Autodesk Inventor part; units mm, degrees
ref_plane "YZ Plane" through (0, 0, 0) normal (1, 0, 0) x (0, 1, 0)
ref_plane "XZ Plane" through (0, 0, 0) normal (0, 1, 0) x (-1, 0, 0)
ref_plane "XY Plane" through (0, 0, 0) normal (0, 0, 1) x (1, 0, 0)
sketch "Sketch1" plane through (0, 0, 0) normal (0, 0, 1) x (1, 0, 0)
  line L0 (32.5, 60) -> (-32.5, 60)
  line L1 (-32.5, 60) -> (-32.5, -60)
  line L2 (-32.5, -60) -> (32.5, -60)
  line L3 (32.5, -60) -> (32.5, 60)
  line L4 (32.5, 60) -> (-32.5, -60) construction
  line L5 (-32.5, 60) -> (32.5, -60) construction
  line L6 (-27, 57) -> (27, 57) construction
  line L7 (27, 57) -> (27, -57) construction
  line L8 (27, -57) -> (-27, -57) construction
  line L9 (-27, -57) -> (-27, 57) construction
  line L10 (-27, 57) -> (27, -57) construction
  line L11 (27, 57) -> (-27, -57) construction
  arc A0 (22.4174, 59) -> (31.5, 54.8206) centre (27, 57) ccw
  line L12 (31.5, 54.8206) -> (31.5, -54.8206)
  line L13 (22.4174, 59) -> (-22.4174, 59)
  line L14 (32.5, 0) -> (-32.5, 0) construction
  line L15 (0, 60) -> (0, -60) construction
  arc A1 (31.5, -54.8206) -> (22.4174, -59) centre (27, -57) ccw
  line L16 (22.4174, -59) -> (-22.4174, -59)
  arc A2 (-31.5, 54.8206) -> (-22.4174, 59) centre (-27, 57) ccw
  line L17 (-31.5, 54.8206) -> (-31.5, -54.8206)
  arc A3 (-22.4174, -59) -> (-31.5, -54.8206) centre (-27, -57) ccw
  point P0 (0, 0)
  dimension "d0" = 65
  dimension "d1" = 120
  dimension "d2" = 5.5
  dimension "d3" = 3
  dimension "d4" = 1
  dimension "d5" = 1
  dimension "d6" = 5
extrude "Extrusion1" add sketch "Sketch1" along normal blind 1.6 contours L3 L2 L1 L0 | A0 L12 A1 L16 A3 L17 A2 L13
extrude "Extrusion2" add sketch "Sketch1" along normal blind 14.1 contours A0 L12 A1 L16 A3 L17 A2 L13
hole "Hole1" at (27, 57, 0) at (-27, 57, 0) at (-27, -57, 0) at (27, -57, 0) direction (0, 0, 1) diameter 3.5 end through all
fillet "Fillet1" radius 2 8 edges at (-22.4174, 59, 7.85) (-31.5, 54.8206, 7.85) (22.4174, 59, 7.85) (31.5, 54.8206, 7.85) (31.5, -54.8206, 7.85) (22.4174, -59, 7.85) (-22.4174, -59, 7.85) (-31.5, -54.8206, 7.85)
equation "\"d5\" = d4"
properties part number "SUSTAINA-CORE-BOARD" material "Acetal Resin, Black"
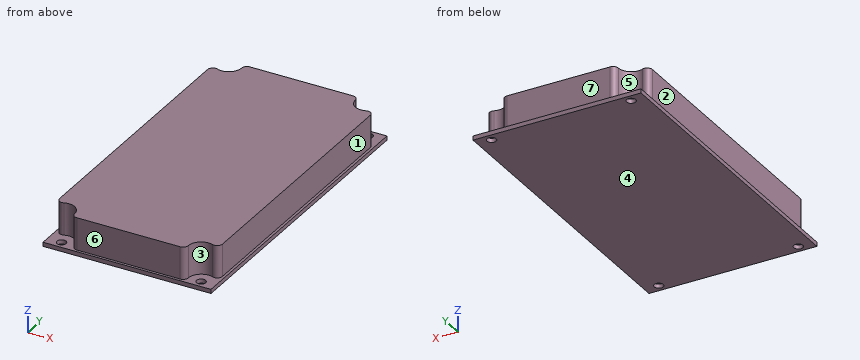
Verification items for the finished model (mm, model axes). Face numbers are marked on the shaded views. A direction names the side the tool comes from. Give positions to 0.01 mm unless a question says otherwise; leave off trailing zeros. Write each loop counter-clockwise with the first axis right and the second up, starting at its lowest first coordinate (ties: lowest second). Pieces come first, ordered by that corner, then holes. Notation, with made-up numbers: M 25.25,26.25 L 77.25,26.25 A10 cw 77.25,33.25 Z; hole C 55,9.25 d8. An arc over 180 degrees is marked long. Use CSV: the item, a comma, the result in double quotes.
1) Release check for a two-part mould opening along X. For the marked faces 1, 2 and 3 record: released by +X, released by -X, zero draft, split by the parting line, or undercut.
Final values:
face 1,"released by +X"
face 2,"released by -X"
face 3,"undercut"
2) Cross-section at A-A (x = -27). Enter the section's corners in (y, z).
Final values:
outline,"M -60,0 L -58.75,0 L -58.75,1.6 L -60,1.6 Z; M -55.25,0 L 55.25,0 L 55.25,1.6 L 52,1.6 L 52,14.1 L -52,14.1 L -52,1.6 L -55.25,1.6 Z; M 58.75,0 L 60,0 L 60,1.6 L 58.75,1.6 Z"
3) Cross-section at B-B (y = 35). Enter the section's corners in (x, z), plus the area to 4 significant figures.
Final values:
outline,"M -32.5,0 L 32.5,0 L 32.5,1.6 L 31.5,1.6 L 31.5,14.1 L -31.5,14.1 L -31.5,1.6 L -32.5,1.6 Z"
area,"891.5 mm²"
4) Go/stop test with flat-tipped pins: pin 1 Ø6 at (y, z) = (45.5, 11) entering from +X; pin 2 Ø5.5 at (x, y) = (-27, -57) entering from +Z; pin 3 Ø1.5 at (x, z) = (9, 11) entering from -Y. Record where each tip stops, or that it passes through.
Final values:
pin 1,"x = 31.5"
pin 2,"z = 1.6"
pin 3,"y = -59"
5) Cross-section at C-C (z = 12.25). Enter the section's corners in (x, y), plus the area to 3 significant figures.
Final values:
outline,"M -31.5,-50.46 A2 ccw -28.79,-52.33 A5 cw -22,-57 A2 ccw -20,-59 L 20,-59 A2 ccw 22,-57 A5 cw 28.79,-52.33 A2 ccw 31.5,-50.46 L 31.5,50.46 A2 ccw 28.79,52.33 A5 cw 22,57 A2 ccw 20,59 L -20,59 A2 ccw -22,57 A5 cw -28.79,52.33 A2 ccw -31.5,50.46 Z"
area,"7,190 mm²"
6) Access from +Z, -Z, +X, -X, +Y, -Y to the whole of each face (thin tool, end or side, straight path). Record for the marked faces 4, 5, 6 and 7.
Final values:
face 4,"-Z, +X, -X, +Y, -Y"
face 5,"+Z, +Y"
face 6,"+Z, +X, -X, -Y"
face 7,"+Z, +X, -X, +Y"
7) Material ranges on line 1 along Y through (x, z) = (-27, 0.8); line 2 along X through (y, z) = (57, 0.7); line 3 along X through (y, z) = (-37, 4.5), recorded low to high.
Final values:
line 1,"-60 to -58.75, -55.25 to 55.25, 58.75 to 60"
line 2,"-32.5 to -28.75, -25.25 to 25.25, 28.75 to 32.5"
line 3,"-31.5 to 31.5"
